Build history of the part. All positions in model axes, mm. Round coordinates to 2 decimals unless told otherwise and drop trailing zeros. Write each loop counter-clockwise with the first axis right and the second up, starting at its lowest first coordinate (ties: lowest second). Pieces come first, ordered by that corner, then holes. Notation, with made-up numbers: M 49.5,71 L 55.5,71 A27 cw 55.5,100 Z; hole C 80.25,81.5 d8. An arc over 180 degrees is marked long. Write item = value, one per line. Start each with the question number.
Q1. Band-saw the part on B-B on y = 12. Write the cut outline in (x, z).
Q2. Drop a flat-ended pin along its axis: P1, Ø3, axis at x = 9, y = 16.5, coming from the +Z side. Give the stop position or say it passes through.
Q3. Band-saw the part on A-A on x = 37. Write the cut outline in (y, z).
Q4. Band-saw the part on C-C on z = -3.75. Write the cut outline in (x, y).
Q5. Probe L1, parallel to Z at x = 27.5, y = 20.75; L2, parallel to Y at x = 45, z = -3; L3, parallel to Z at x = 18.5, y = 16.75. List the from-to ranges inside material, lowest first.
```python
from build123d import *

# Parameters (mm, degrees)
SKETCH1_W            = 48
SKETCH1_H            = 53
BOSS_EXTRUDE1_DEPTH  = 10
SKETCH2_W            = 48
SKETCH2_H            = 5.616325
BOSS_EXTRUDE2_DEPTH  = 33.1917878
SKETCH4_W            = 4
SKETCH4_H            = 10
BOSS_EXTRUDE4_DEPTH  = 40
SKETCH5_W            = 48
SKETCH5_H            = 10.8609375
BOSS_EXTRUDE5_DEPTH  = 23.1917878
SKETCH6_W            = 48
SKETCH6_H            = 5
BOSS_EXTRUDE6_DEPTH  = 42.3
SKETCH7_W            = 12.8082122
SKETCH7_H            = 16.4772625
BOSS_EXTRUDE7_DEPTH  = 48
CUT_EXTRUDE1_REACH   = 84.426
SKETCH8_R            = 11.5
SKETCH8_R_2          = 2
FILLET1_R            = 10
FILLET2_R            = 4
SKETCH9_W            = 5
SKETCH9_H            = 16.4772625
BOSS_EXTRUDE9_DEPTH  = 48
CUT_EXTRUDE2_DEPTH   = 6
SKETCH11_R           = 1.9304
CUT_EXTRUDE3_DEPTH   = 6
BOSS_EXTRUDE11_DEPTH = 3
BOSS_EXTRUDE12_DEPTH = 48
SKETCH14_W           = 119.824941969
SKETCH14_H           = 122.237524693
CUT_EXTRUDE4_DEPTH   = 90.10667764
SKETCH15_W           = 48
SKETCH15_H           = 17.1390625
BOSS_EXTRUDE13_DEPTH = 3.175


with BuildPart() as part:
    # Sketch1 → Boss-Extrude1 (new body)
    with BuildSketch(Plane.XY):
        with Locations((24, 26.5)):
            Rectangle(SKETCH1_W, SKETCH1_H)
    extrude(amount=BOSS_EXTRUDE1_DEPTH)

    # Sketch2 → Boss-Extrude2 (add)
    with BuildSketch(Plane(origin=(0, 0, 0), x_dir=(-1, 0, 0), z_dir=(0, 0, -1))):
        with Locations((-24, -2.8081625)):
            Rectangle(SKETCH2_W, SKETCH2_H)
    extrude(amount=-BOSS_EXTRUDE2_DEPTH)

    # Sketch4 → Boss-Extrude4 (add)
    with BuildSketch(Plane.XY.offset(10)):
        with Locations((2, 48)):
            Rectangle(SKETCH4_W, SKETCH4_H)
        with Locations((46, 48)):
            Rectangle(SKETCH4_W, SKETCH4_H)
    extrude(amount=BOSS_EXTRUDE4_DEPTH)

    # Sketch5 → Boss-Extrude5 (add)
    with BuildSketch(Plane.XY.offset(10)):
        with Locations((24, 5.43046875)):
            Rectangle(SKETCH5_W, SKETCH5_H)
    extrude(amount=BOSS_EXTRUDE5_DEPTH)

    # Sketch6 → Boss-Extrude6 (add)
    with BuildSketch(Plane.XZ.offset(5.616325)):
        with Locations((24, 30.6917878)):
            Rectangle(SKETCH6_W, SKETCH6_H)
    extrude(amount=BOSS_EXTRUDE6_DEPTH)

    # Sketch7 → Boss-Extrude7 (add)
    with BuildSketch(Plane.ZY):
        with Locations((-6.4041061, 2.62230625)):
            Rectangle(SKETCH7_W, SKETCH7_H)
    extrude(amount=-BOSS_EXTRUDE7_DEPTH)

    # Sketch8 → Cut-Extrude1 (cut, up to next)
    with BuildSketch(Plane(origin=(0, 0, 28.1917878), x_dir=(-1, 0, 0), z_dir=(0, 0, -1)), mode=Mode.PRIVATE) as cut_extrude1_sk1:
        with Locations((-24, -26.616325)):
            Circle(SKETCH8_R)
    cut_extrude1_tool1 = extrude(cut_extrude1_sk1.sketch, amount=-CUT_EXTRUDE1_REACH, mode=Mode.PRIVATE) & part.part
    # Sketch8 → Cut-Extrude1 (cut, up to next)
    with BuildSketch(Plane(origin=(0, 0, 28.1917878), x_dir=(-1, 0, 0), z_dir=(0, 0, -1)), mode=Mode.PRIVATE) as cut_extrude1_sk2:
        with Locations((-39.5, -11.116325)):
            Circle(SKETCH8_R_2)
    cut_extrude1_tool2 = extrude(cut_extrude1_sk2.sketch, amount=-CUT_EXTRUDE1_REACH, mode=Mode.PRIVATE) & part.part
    # Sketch8 → Cut-Extrude1 (cut, up to next)
    with BuildSketch(Plane(origin=(0, 0, 28.1917878), x_dir=(-1, 0, 0), z_dir=(0, 0, -1)), mode=Mode.PRIVATE) as cut_extrude1_sk3:
        with Locations((-39.5, -42.116325)):
            Circle(SKETCH8_R_2)
    cut_extrude1_tool3 = extrude(cut_extrude1_sk3.sketch, amount=-CUT_EXTRUDE1_REACH, mode=Mode.PRIVATE) & part.part
    # Sketch8 → Cut-Extrude1 (cut, up to next)
    with BuildSketch(Plane(origin=(0, 0, 28.1917878), x_dir=(-1, 0, 0), z_dir=(0, 0, -1)), mode=Mode.PRIVATE) as cut_extrude1_sk4:
        with Locations((-8.5, -11.116325)):
            Circle(SKETCH8_R_2)
    cut_extrude1_tool4 = extrude(cut_extrude1_sk4.sketch, amount=-CUT_EXTRUDE1_REACH, mode=Mode.PRIVATE) & part.part
    # Sketch8 → Cut-Extrude1 (cut, up to next)
    with BuildSketch(Plane(origin=(0, 0, 28.1917878), x_dir=(-1, 0, 0), z_dir=(0, 0, -1)), mode=Mode.PRIVATE) as cut_extrude1_sk5:
        with Locations((-8.5, -42.116325)):
            Circle(SKETCH8_R_2)
    cut_extrude1_tool5 = extrude(cut_extrude1_sk5.sketch, amount=-CUT_EXTRUDE1_REACH, mode=Mode.PRIVATE) & part.part
    add(cut_extrude1_tool1.solids().sort_by_distance((24, -26.616325, 28.191788))[0], mode=Mode.SUBTRACT)
    add(cut_extrude1_tool2.solids().sort_by_distance((39.5, -11.116325, 28.191788))[0], mode=Mode.SUBTRACT)
    add(cut_extrude1_tool3.solids().sort_by_distance((39.5, -42.116325, 28.191788))[0], mode=Mode.SUBTRACT)
    add(cut_extrude1_tool4.solids().sort_by_distance((8.5, -11.116325, 28.191788))[0], mode=Mode.SUBTRACT)
    add(cut_extrude1_tool5.solids().sort_by_distance((8.5, -42.116325, 28.191788))[0], mode=Mode.SUBTRACT)

    # Fillet1
    fillet1_edges = [part.edges().sort_by_distance(p)[0] for p in [
        (24, 10.8609375, 0),
    ]]
    fillet(fillet1_edges, radius=FILLET1_R)

    # Fillet2
    fillet2_edges = [part.edges().sort_by_distance(p)[0] for p in [
        (2, 43, 10),
        (46, 43, 10),
    ]]
    fillet(fillet2_edges, radius=FILLET2_R)

    # Sketch9 → Boss-Extrude9 (add)
    with BuildSketch(Plane(origin=(48, 0, 0), x_dir=(0, 0, -1), z_dir=(1, 0, 0))):
        with Locations((15.3082122, 2.62230625)):
            Rectangle(SKETCH9_W, SKETCH9_H)
    extrude(amount=-BOSS_EXTRUDE9_DEPTH)

    # Sketch10 → Cut-Extrude2 (cut)
    with BuildSketch(Plane.XY.offset(10)):
        Polygon((12.429, 36.979734073), (9, 38.959468146), (5.571, 36.979734073), (5.571, 33.020265927), (9, 31.040531854), (12.429, 33.020265927), align=None)
        Polygon((35.571, 36.979734073), (35.571, 33.020265927), (39, 31.040531854), (42.429, 33.020265927), (42.429, 36.979734073), (39, 38.959468146), align=None)
    extrude(amount=-CUT_EXTRUDE2_DEPTH, mode=Mode.SUBTRACT)

    # Sketch11 → Cut-Extrude3 (cut)
    with BuildSketch(Plane.XY.offset(4)):
        with Locations((9, 35)):
            Circle(SKETCH11_R)
        with Locations((39, 35)):
            Circle(SKETCH11_R)
    extrude(amount=-CUT_EXTRUDE3_DEPTH, mode=Mode.SUBTRACT)

    # Sketch12 → Boss-Extrude11 (add)
    with BuildSketch(Plane(origin=(0, 53, 0), x_dir=(1, 0, 0), z_dir=(0, 1, 0))):
        Polygon((0, 0), (0, -50), (4, -50), (4, -10), (44, -10), (44, -50), (48, -50), (48, 0), align=None)
    extrude(amount=BOSS_EXTRUDE11_DEPTH)

    # Sketch13 → Boss-Extrude12 (add)
    with BuildSketch(Plane(origin=(48, 0, 0), x_dir=(0, 0, -1), z_dir=(1, 0, 0))):
        with BuildLine():
            Line((17.8082122, 10.8609375), (10, 10.8609375))
            ThreePointArc((10, 10.8609375), (2.928932188, 13.789869688), (0, 20.8609375))
            Line((0, 20.8609375), (0, 28))
            Line((0, 28), (17.8082122, 28))
            Line((17.8082122, 28), (17.8082122, 10.8609375))
        make_face()
    extrude(amount=-BOSS_EXTRUDE12_DEPTH)

    # Sketch14 → Cut-Extrude4 (cut, through all)
    with BuildSketch(Plane(origin=(48, 0, 0), x_dir=(0, 0, -1), z_dir=(1, 0, 0))):
        with Locations((-16.90365686, 8.216937598)):
            Rectangle(SKETCH14_W, SKETCH14_H)
        with BuildLine():
            Line((0, 28), (0, 20.8609375))
            ThreePointArc((0, 20.8609375), (2.928932188, 13.789869688), (10, 10.8609375))
            Line((10, 10.8609375), (17.8082122, 10.8609375))
            Line((17.8082122, 10.8609375), (17.8082122, 28))
            Line((17.8082122, 28), (0, 28))
        make_face(mode=Mode.SUBTRACT)
    extrude(amount=-CUT_EXTRUDE4_DEPTH, mode=Mode.SUBTRACT)

    # Sketch15 → Boss-Extrude13 (add)
    with BuildSketch(Plane(origin=(0, 0, -17.8082122), x_dir=(-1, 0, 0), z_dir=(0, 0, -1))):
        with Locations((-24, 19.43046875)):
            Rectangle(SKETCH15_W, SKETCH15_H)
    extrude(amount=BOSS_EXTRUDE13_DEPTH)


solid = part.part
```
Conclusion:
q1.outline = M 0,-20.98 L 48,-20.98 L 48,-5.36 L 0,-5.36 Z
q2.P1 = -0.42
q3.outline = M 10.86,-20.98 L 28,-20.98 L 28,0 L 20.86,0 A10 ccw 10.86,-10 Z
q4.outline = M 0,13.05 L 48,13.05 L 48,28 L 0,28 Z
q5.L1 = -20.98 to 0
q5.L2 = 13.72 to 28
q5.L3 = -20.98 to -0.88
